from build123d import *

# Parameters (mm, degrees)
F0_W     = 6
F0_H     = 0.3
F1_DEPTH = 2.5
F2_R     = 2


# Not quite as in the source:
# - a feature names something its author has since deleted; it is built from what else it names


with BuildPart() as f1:
    # F0 (on Top) → F1 (new body)
    with BuildSketch(Plane.XY):
        Polygon((3.5, 0), (-3.5, 0), (-3.5, -65), (-23.5, -65), (-23.5, -70), (-17.5, -70), (-1.25, -70), (-1.25, -55), (1.25, -55), (1.25, -70), (17.5, -70), (23.5, -70), (23.5, -65), (3.5, -65), align=None)
        with Locations((-20.5, -70.15)):
            Rectangle(F0_W, F0_H)
        with Locations((20.5, -70.15)):
            Rectangle(F0_W, F0_H)
        Polygon((-40, 40), (-40, 0), (-3.5, 0), (3.5, 0), (40, 0), (40, 40), align=None)
    extrude(amount=F1_DEPTH)

    # F2
    f2_edges = [f1.edges().sort_by_distance(p)[0] for p in [
        (-3.5, 0, 1.25),
        (3.5, 0, 1.25),
        (3.5, -65, 1.25),
        (-3.5, -65, 1.25),
        (-23.5, -65, 1.25),
        (23.5, -65, 1.25),
        (-23.5, -70.3, 1.25),
        (23.5, -70.3, 1.25),
        (40, 0, 1.25),
        (-40, 0, 1.25),
    ]]
    fillet(f2_edges, radius=F2_R)


solid = f1.part
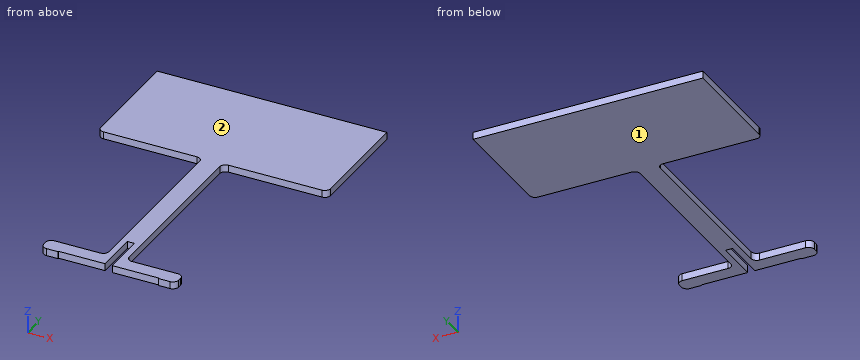
CAD build for the part. Positions are in the model's coordinates, mm. Face numbers are marked on the shaded views. Coordinates: 2 decimals unless noted, no trailing zeros. Order: outer loops, then holes, each group sorted by start corner. A loop starts at its lowest first (then second) coordinate and runs counter-clockwise, first axis right, second up.
Item 1: Pin check, flat tips, straight feed: pin 1 Ø1.2 at (y, z) = (-30, 0.5) entering from +X; pin 2 Ø1.2 at (x, z) = (0, 1) entering from -Y; pin 3 Ø0.7 at (y, z) = (-68, 1.5) entering from -X; pin 4 Ø10 at (x, y) = (4, -23.5) entering from -Z. Stop position of each tip, or through.
Check sheet entries:
pin 1: stops at x = 3.5
pin 2: stops at y = -55
pin 3: stops at x = -23.5
pin 4: stops at z = 0
Item 2: Band-saw the part on A-A on x = -16. List the corners of the cut face in (y, z), plus the area to 4 significant figures.
Check sheet entries:
outline: (-70, 0) - (-65, 0) - (-65, 2.5) - (-70, 2.5) - close; (0, 0) - (40, 0) - (40, 2.5) - (0, 2.5) - close
area: 112.5 mm2
Item 3: Band-saw the part on C-C on y = -11. List the corners of the cut face in (x, z).
Check sheet entries:
outline: (-3.5, 0) - (3.5, 0) - (3.5, 2.5) - (-3.5, 2.5) - close
Item 4: Drill centre lines: L1, parallel to X at y = -58.5, z = 0.95; L2, parallel to Y at x = 18.5, z = 1.85; L3, parallel to Y at x = 6, z = 1.4. Where is each one in solid material? Low to high.
Check sheet entries:
L1: x = -3.5 to -1.25, 1.25 to 3.5
L2: y = -70.3 to -65, 0 to 40
L3: y = -70 to -65, 0 to 40
Item 5: Band-saw the part on D-D on x = 28. List the corners of the cut face in (y, z), plus the area to 3 significant figures.
Check sheet entries:
outline: (0, 0) - (40, 0) - (40, 2.5) - (0, 2.5) - close
area: 100 mm2
Item 6: Two-plate mould, pull along Z, no slides. Class the marked faces 1 and 2: +Z half, -Z half, draft (parallel to the pull), parting line (faces both ways), or undercut.
Check sheet entries:
face 1: -Z half
face 2: +Z half
